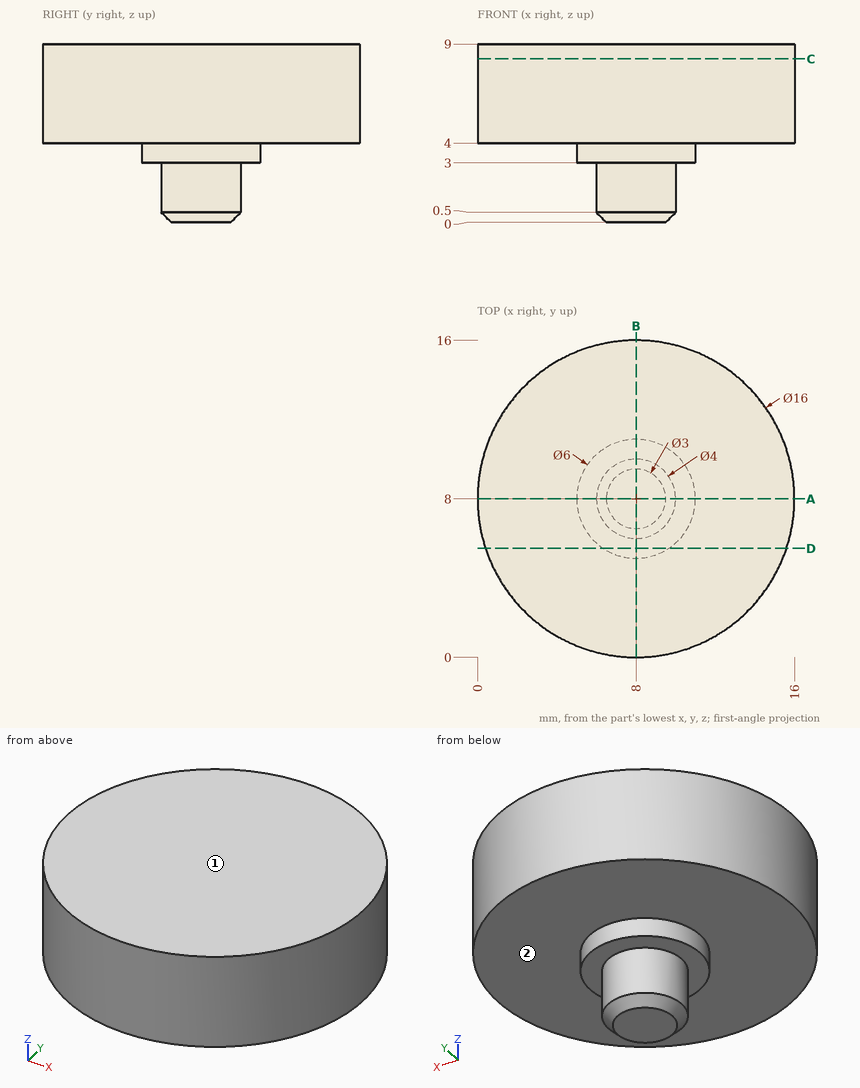
Source: three-view drawing plus pictorial views. Frame: mm from the lowest corner of the part. A direction names the side the tool comes from. Round coordinates to 2 decimals unless told otherwise and drop trailing zeros. Loops run counter-clockwise (first coordinate to the right, second up) from the corner with the lowest first, then second, coordinate; pieces in that order, holes last. Notation, with made-up numbers: M 25.5,47 L 70.5,47 A17 cw 70.5,57 Z; hole C 43.25,-4.5 d1. An arc over 180 degrees is marked long. Answer as CSV lines item,"result". Start each with the question number.
(1) Section D-D, the plane y = 5.5. Output: boundary loops of the cut face in (x, z), plus the area to 3 significant figures.
(2) Reachability of the marked faces 1 and 2 from +Z, -Z, +X, -X, +Y, -Y: full face, straight path, thin tool, end or side. Return the list, or none.
(3) First-contact query: pin 1 (1 mm diameter, centred on x = 10, z = 1, fed in from +Y); pin 2 (1.5 mm diameter, centred on y = 11.5, z = 8, fed in from -X); pin 3 (1 mm diameter, centred on y = 5, z = 5.5, fed in from -X). Flat tips, straight axial feed; report the tip coordinate or a pass-through.
(4) Section C-C, the plane z = 8.25. Output: boundary loops of the cut face in (x, y), plus the area to 3 significant figures.
(5) Line query: line 1 (Z direction, x = 1, y = 9.75); line 2 (Z direction, x = 10.5, y = 6.5); line 3 (X direction, y = 9.5, z = 6.75). Output: solid intervals per line, ascending. Write a range as [from, to].
(6) Section A-A, the plane y = 8. Output: boundary loops of the cut face in (x, z), plus the area to 4 significant figures.
Values found:
1,outline,"M 0.4,4 L 6.34,4 L 6.34,3 L 9.66,3 L 9.66,4 L 15.6,4 L 15.6,9 L 0.4,9 Z"
1,area,"79.3 mm²"
2,face 1,"+Z, +X, -X, +Y, -Y"
2,face 2,"-Z"
3,pin 1,"stops at y = 9.32"
3,pin 2,"stops at x = 0.49"
3,pin 3,"stops at x = 0.4"
4,outline,"C 8,8 d16"
4,area,"201 mm²"
5,line 1,"z = [4, 9]"
5,line 2,"z = [3, 9]"
5,line 3,"x = [0.14, 15.86]"
6,outline,"M 0,4 L 5,4 L 5,3 L 6,3 L 6,0.5 L 6.5,0 L 9.5,0 L 10,0.5 L 10,3 L 11,3 L 11,4 L 16,4 L 16,9 L 0,9 Z"
6,area,"97.75 mm²"
